Geometry: final body of the model. Coordinates: model frame, mm. Give positions to 0.01 mm unless a question says otherwise; leave off trailing zeros. Write each loop counter-clockwise with the first axis right and the second up, starting at its lowest first coordinate (ties: lowest second). Pieces come first, ordered by that corner, then holes. Notation, with made-up numbers: M -38,6 L -10,6 A27 cw -10,27 Z; hole C 8.25,-21.5 d11. An arc over 180 degrees is marked long. Use one line per item in the form item = value. Start each with the question number.
Item 1: Section query C-C on x = -3. Return loops of the section in (y, z), then the cut area to 3 significant figures.
Item 2: Contact query for flat-ended pins moving along their axis: P1, Ø4, axis at y = -4, z = -2, coming from the +X side; P2, Ø6, axis at y = 0, z = -3.5, coming from the +X side; P3, Ø6, axis at x = 1, y = -3.5, coming from the -Z side. Output: stop coordinate, or through.
Item 3: Pull-direction query (Y, two-part tool) for faces 1 (the cylindrical face through (0.11, -4.88, 1.08)), 2 (the cylindrical face through (0.105, -0.867, -3.905)); classes: released by +Y, released by -Y, zero draft, split by the parting line, or undercut.
Item 4: Section query D-D on z = 4.25. Return loops of the section in (x, y).
Item 5: Material intervals for line 1 along Z through (x, y) = (-2.5, 3); line 2 along Z through (x, y) = (-6.25, -0.25); line 3 along Y through (x, z) = (5, 1.75), sorted ascending. Write a range as from..to.
Item 6: Section query A-A on y = 0. Return loops of the section in (x, z).
from build123d import *

# Parameters (mm, degrees)
SKETCH1_R           = 5
BOSS_EXTRUDE1_DEPTH = 7.5
DOME1_FACE_RADIUS   = 5
DOME1_HEIGHT        = 5


# Read off the part's stored shape, not the designer's step: Shell1
with BuildPart() as part:
    # Sketch1 → Boss-Extrude1 (new, symmetric)
    with BuildSketch(Plane(origin=(0, 0, 0), x_dir=(0, 0, -1), z_dir=(1, 0, 0))):
        Circle(SKETCH1_R)
    extrude(amount=BOSS_EXTRUDE1_DEPTH, both=True)

    # Dome1: a dome of height H over a round flat face of radius A is a cap of a sphere of radius (A * A + H * H) / (2 * H)
    dome1_r = (DOME1_FACE_RADIUS * DOME1_FACE_RADIUS + DOME1_HEIGHT * DOME1_HEIGHT) / (2 * DOME1_HEIGHT)
    dome1_base = Plane((7.5, 0, 0), z_dir=(1, 0, 0))
    with Locations(dome1_base.offset(DOME1_HEIGHT - dome1_r)):
        dome1_ball = Sphere(dome1_r, mode=Mode.PRIVATE)
    add(split(dome1_ball, bisect_by=dome1_base, keep=Keep.TOP, mode=Mode.PRIVATE))

    # Shell1 outline → Shell1 (revolve, cut)
    with BuildSketch(Plane.YX):
        with BuildLine():
            Line((4, -7.5), (4, 7.499999996))
            ThreePointArc((4, 7.499999996), (2.828427126, 10.328427123), (0, 11.5))
            Line((0, 11.5), (0, -7.5))
            Line((0, -7.5), (4, -7.5))
        make_face()
    revolve(axis=Axis((0, 0, 0), (1, 0, 0)), mode=Mode.SUBTRACT)


solid = part.part
Answer sheet:
q1.outline = C 0,0 d10; hole C 0,0 d8
q1.area = 28.3 mm2
q2.P1 = 11.85
q2.P2 = 12.47
q2.P3 = -4.97
q3.face_1 = split by the parting line
q3.face_2 = undercut
q4.outline = M -7.5,-2.63 L 7.5,-2.63 A2.63 ccw 7.5,2.63 L -7.5,2.63 Z
q5.line_1 = -4..-2.65, 2.65..4
q5.line_2 = -4.99..-3.99, 3.99..4.99
q5.line_3 = -4.68..-3.6, 3.6..4.68
q6.outline = M -7.5,-5 L 7.5,-5 A5 ccw 7.5,5 L -7.5,5 L -7.5,4 L 7.5,4 A4 cw 7.5,-4 L -7.5,-4 Z
